from build123d import *

# Parameters (mm, degrees)
BOSS_EXTRUDE1_DEPTH     = 10
CUT_EXTRUDE1_DEPTH      = 234.65368604
CUT_EXTRUDE1_DEPTH_BACK = 234.65368604
SKETCH3_R               = 4
FILLET1_R               = 4
FILLET2_R               = 4


with BuildPart() as part:
    # Sketch1 → Revolve1 (revolve)
    with BuildSketch(Plane.XY):
        Polygon((0, 0), (-7.9, 0), (-7.9, 200), (-12.35, 200), (-12.35, 233), (-4.35, 233), (-4.35, 220), (0, 220), align=None)
    revolve(axis=Axis((0, 220, 0), (0, -1, 0)))

    # Sketch2 → Boss-Extrude1 (add)
    with BuildSketch(Plane(origin=(0, 220, 0), x_dir=(1, 0, 0), z_dir=(0, 1, 0))):
        with BuildLine():
            ThreePointArc((4.35, 0), (3.817394399, 2.085665361), (2.35, 3.660601044))
            Line((2.35, 3.660601044), (2.35, -3.660601044))
            ThreePointArc((2.35, -3.660601044), (3.817394399, -2.085665361), (4.35, 0))
        make_face()
    extrude(amount=BOSS_EXTRUDE1_DEPTH)

    # Sketch3 → Cut-Extrude1 (cut, two sides: drawn at the far end of the back side and taken through both)
    with BuildSketch(Plane(origin=(0, 0, 0), x_dir=(0, 0, -1), z_dir=(1, 0, 0)).offset(-CUT_EXTRUDE1_DEPTH_BACK)):
        with Locations((0, 20)):
            Circle(SKETCH3_R)
    extrude(amount=CUT_EXTRUDE1_DEPTH + CUT_EXTRUDE1_DEPTH_BACK, mode=Mode.SUBTRACT)

    # Fillet1
    fillet1_edges = [part.edges().sort_by_distance(p)[0] for p in [
        (12.35, 200, 0),
    ]]
    fillet(fillet1_edges, radius=FILLET1_R)

    # Fillet2
    fillet2_edges = [part.edges().sort_by_distance(p)[0] for p in [
        (7.9, 200, 0),
    ]]
    fillet(fillet2_edges, radius=FILLET2_R)


solid = part.part
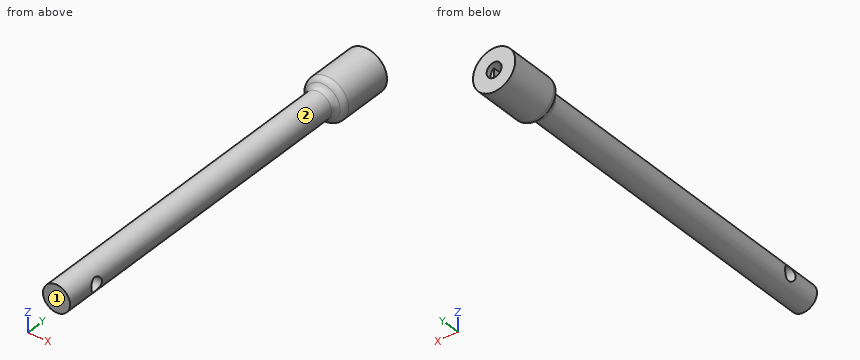
Geometry: final body of the model. Coordinates: model frame, mm. Face numbers are marked on the shaded views. A direction names the side the tool comes from. Round coordinates to 2 decimals unless told otherwise and drop trailing zeros. Order: outer loops, then holes, each group sorted by start corner. A loop starts at its lowest first (then second) coordinate and runs counter-clockwise, first axis right, second up. Notation, with made-up numbers: (37, -39) -> (87, -39) arc R7 ccw to (87, -32) -> close; hole circle Ø1 at (-17.75, 3). An arc over 180 degrees is marked (long way). Put each result on its own line as item: value. Start each with the question number.
Q1. Section A-A on y = 207.5. Return the cut outline in (x, z), and give its area (3 significant figures).
Q2. Reachability of the marked faces 1 and 2 from +Z, -Z, +X, -X, +Y, -Y: full face, straight path, thin tool, end or side. Return the list, or none.
Q3. Line query: probe 1 along Z at (x, y) = (-0.75, 20); probe 2 along Y at (x, z) = (-4.5, 0); probe 3 along Y at (x, z) = (-1.75, 0). Output: solid intervals per line, ascending.
Q4. First-contact query: pin 1 (10 mm diameter, centred on x = 0, z = 0, fed in from +Y); pin 2 (10 mm diameter, centred on x = 1.5, y = 96, fed in from -Z); pin 3 (10.5 mm diameter, centred on y = 20, z = 0, fed in from +X); pin 4 (4 mm diameter, centred on x = 6, y = 89, fed in from +Z). Flat tips, straight axial feed; report the tip coordinate or a pass-through.
Q5. Section B-B on y = 20. Return the cut outline in (x, z).
Q6. Section C-C on y = 116.5. Return the cut outline in (x, z), and give its area (3 significant figures).
Ans:
1. outline: circle Ø24.7 at (0, 0)
1. area: 479 mm2
2. face 1: +Z, -Z, +X, -X, -Y
2. face 2: -Y
3. probe 1: z = -7.86 to -4, 4 to 7.86
3. probe 2: y = 0 to 16, 24 to 233
3. probe 3: y = 0 to 16, 24 to 220
4. pin 1: stops at y = 233
4. pin 2: stops at z = -7.9
4. pin 3: stops at x = 7.9
4. pin 4: stops at z = 6.81
5. outline: (-6.81, -4) arc R7.9 ccw to (6.81, -4) -> close; (-6.81, 4) -> (6.81, 4) arc R7.9 ccw to start
6. outline: circle Ø15.8 at (0, 0)
6. area: 196 mm2
